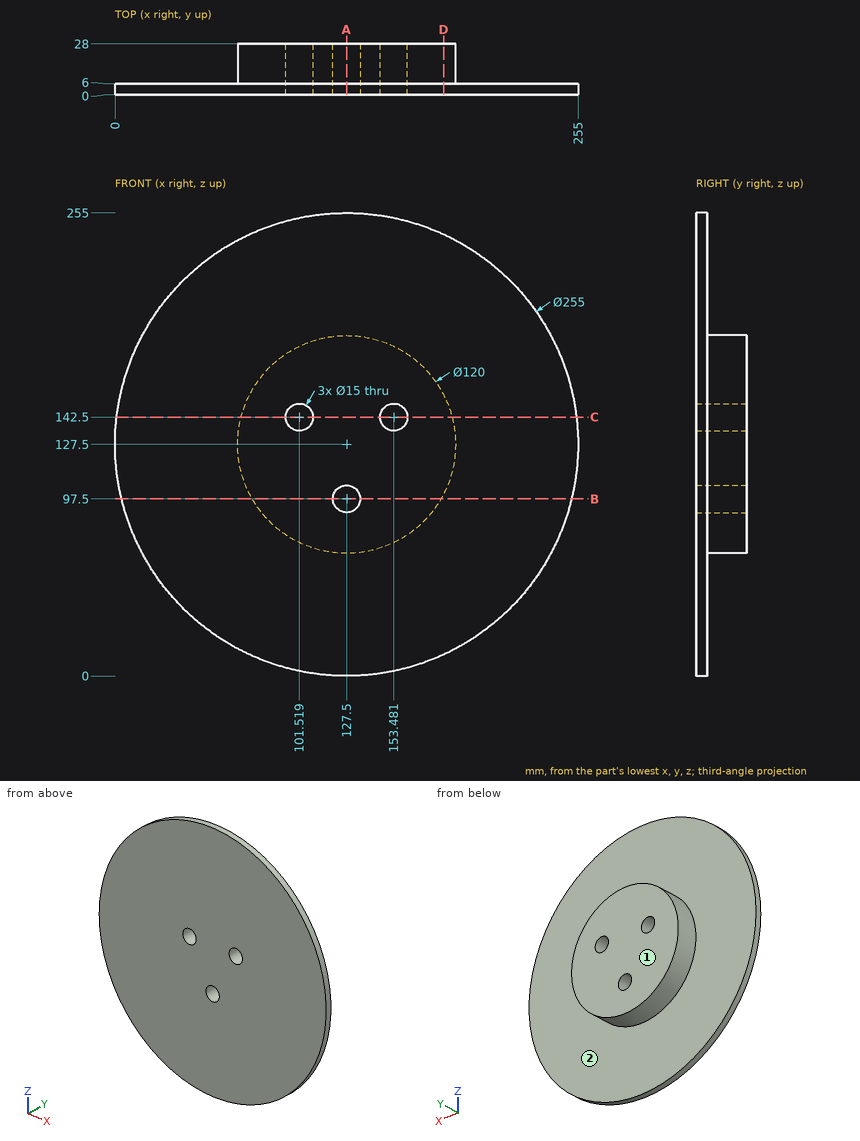
Can you work these out from the drawing? Everything is in mm from the part's minimum corner. A direction names the side the tool comes from. Coordinates: 2 decimals unless noted, no trailing zeros. Loops run counter-clockwise (first coordinate to the right, second up) from the corner with the lowest first, then second, coordinate; pieces in that order, holes last. Notation, with made-up numbers: M -29.5,-33.75 L 20.5,-33.75 A28 ccw 20.5,2.25 Z; hole C -18.5,-38.75 d1. An arc over 180 degrees is marked long. One line per item, written item: value.
1. Imagine slicing it at C-C (z = 142.5). List the corners of the cut face in (x, y) for me (1 decimal), and give its area (3 significant figures).
Geometry says:
outline: M 0.9,0 L 94,0 L 94,28 L 69.4,28 L 69.4,6 L 0.9,6 Z; M 109,0 L 146,0 L 146,28 L 109,28 Z; M 161,0 L 254.1,0 L 254.1,6 L 185.6,6 L 185.6,28 L 161,28 Z
area: 3,240 mm2
2. Imagine slicing it at B-B (z = 97.5). List the corners of the cut face in (x, y) for me, and give its area (3 significant figures).
Geometry says:
outline: M 3.58,0 L 120,0 L 120,28 L 75.54,28 L 75.54,6 L 3.58,6 Z; M 135,0 L 251.42,0 L 251.42,6 L 179.46,6 L 179.46,28 L 135,28 Z
area: 3,350 mm2
3. Please list where these lines run through material, in increasing order: probe 1 along Z at (x, y) = (127.5, 15); probe 2 along Y at (x, z) = (171.5, 26.5); probe 3 along Z at (x, y) = (154.5, 5).
Geometry says:
probe 1: z = 67.5 to 90, 105 to 187.5
probe 2: y = 0 to 6
probe 3: z = 2.89 to 135.07, 149.93 to 252.11
4. Imagine slicing it at A-A (x = 127.5). List the corners of the cut face in (y, z) for me, and give its area (3 significant figures).
Geometry says:
outline: M 0,0 L 6,0 L 6,67.5 L 28,67.5 L 28,90 L 0,90 Z; M 0,105 L 28,105 L 28,187.5 L 6,187.5 L 6,255 L 0,255 Z
area: 3,750 mm2
5. Will these pins go through, and if not, where does the flat tip stop? pin 1 Ø1.5 at (y, z) = (11.5, 157.5) entering from +X; pin 2 Ø12 at (x, y) = (199, 10.5) entering from +Z; pin 3 Ø1 at (x, y) = (79, 17) entering from -Z; pin 4 Ø9 at (x, z) = (127.5, 97.5) entering from +Y.
Geometry says:
pin 1: stops at x = 179.89
pin 2: stops at z = 235.65
pin 3: stops at z = 91.5
pin 4: passes through
6. Imagine slicing it at D-D (x = 181). List the corners of the cut face in (y, z) for me, and give its area (3 significant figures).
Geometry says:
outline: M 0,11.77 L 6,11.77 L 6,100.34 L 28,100.34 L 28,154.66 L 6,154.66 L 6,243.23 L 0,243.23 Z
area: 2,580 mm2
7. On a 3-axis mill with a long thin cutter (end or side, diameter ignored), from which of +Z, -Z, +X, -X, +Y, -Y can I reach the whole of each face in a straight line? I mean the marked faces 1 and 2. Say none if no direction works.
Geometry says:
face 1: +Z, -Z, +X, -X, +Y
face 2: +Y
